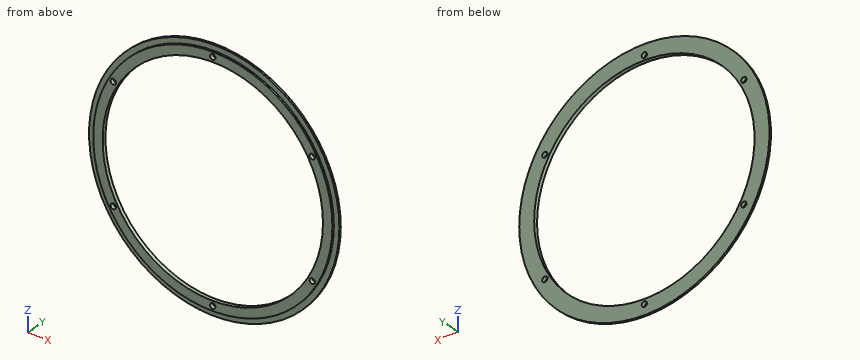
```python
from build123d import *

# Parameters (mm, degrees)
SKETCH1_R           = 160.85
SKETCH1_R_2         = 3.556
SKETCH1_R_3         = 148.15
BOSS_EXTRUDE1_DEPTH = 5.08
SKETCH2_R           = 168.275
SKETCH2_R_2         = 160.85
BOSS_EXTRUDE2_DEPTH = 2.54


with BuildPart() as part:
    # Sketch1 → Boss-Extrude1 (new body)
    with BuildSketch(Plane(origin=(0, 0, 0), x_dir=(1, 0, 0), z_dir=(0, 1, 0))):
        Circle(SKETCH1_R)
        with Locations((0, 154.5)):
            Circle(SKETCH1_R_2, mode=Mode.SUBTRACT)
        with Locations((133.800924885, 77.25)):
            Circle(SKETCH1_R_2, mode=Mode.SUBTRACT)
        with Locations((133.800924885, -77.25)):
            Circle(SKETCH1_R_2, mode=Mode.SUBTRACT)
        with Locations((0, -154.5)):
            Circle(SKETCH1_R_2, mode=Mode.SUBTRACT)
        with Locations((-133.800924885, -77.25)):
            Circle(SKETCH1_R_2, mode=Mode.SUBTRACT)
        with Locations((-133.800924885, 77.25)):
            Circle(SKETCH1_R_2, mode=Mode.SUBTRACT)
        Circle(SKETCH1_R_3, mode=Mode.SUBTRACT)
    extrude(amount=BOSS_EXTRUDE1_DEPTH)

    # Sketch2 → Boss-Extrude2 (add)
    with BuildSketch(Plane(origin=(0, 5.08, 0), x_dir=(1, 0, 0), z_dir=(0, 1, 0))):
        Circle(SKETCH2_R)
        Circle(SKETCH2_R_2, mode=Mode.SUBTRACT)
    extrude(amount=-BOSS_EXTRUDE2_DEPTH)


solid = part.part
```
Can you work these out from the model? Positions are in its coordinate system, mm. Round coordinates to 2 decimals unless told otherwise and drop trailing zeros. Order: outer loops, then holes, each group sorted by start corner. A loop starts at its lowest first (then second) coordinate and runs counter-clockwise, first axis right, second up. Notation, with made-up numbers: (48.5, -31) -> (61.5, -31) arc R29 ccw to (61.5, 0) -> close; hole circle Ø1 at (52, -0.5). An arc over 180 degrees is marked (long way). Return JSON: item names as keys, results as strings. Group by question number.
1. I need wall thicknesses on line 1 (Z direction, x = 0, y = 1.1); line 2 (X direction, y = 1.6, z = -77.25); line 3 (Z direction, x = -134.5, y = 0.75). Which ranges of each line are inside material? Lowest first, please. Write a range as [from, to].
2. If we section it at B-B, the plane y = 3.4: Write out the boundary of the cut face in (x, z) (3 decimals), then the cut area to 3 significant figures.
3. If we section it at C-C, the plane x = -108: Write out the boundary of the cut face in (y, z), then the cut area to 3 significant figures.
4. Will these pins go through, and if not, where does the flat tip stop? pin 1 (2 mm diameter, centred on x = 49, y = 2, fed in from +Z); pin 2 (3 mm diameter, centred on x = 126.5, y = 3.5, fed in from +Z).
5. If we section it at A-A, the plane z = 0: Write out the boundary of the cut face in (x, y) (3 decimals).
Output values:
{
 "1": {"line 1": "[-160.85, -158.06], [-150.94, -148.15], [148.15, 150.94], [158.06, 160.85]", "line 2": "[-141.09, -137.36], [-130.24, -126.42], [126.42, 130.24], [137.36, 141.09]", "line 3": "[-88.22, -80.74], [-73.76, -62.11], [62.11, 73.76], [80.74, 88.22]"},
 "2": {"outline": "circle Ø336.55 at (0, 0); hole circle Ø296.3 at (0, 0); hole circle Ø7.112 at (-133.801, -77.25); hole circle Ø7.112 at (-133.801, 77.25); hole circle Ø7.112 at (0, -154.5); hole circle Ø7.112 at (0, 154.5); hole circle Ø7.112 at (133.801, -77.25); hole circle Ø7.112 at (133.801, 77.25)", "area": "19,800 mm²"},
 "3": {"outline": "(0, -119.2) -> (2.54, -119.2) -> (2.54, -129.04) -> (5.08, -129.04) -> (5.08, -101.41) -> (0, -101.41) -> close; (0, 101.41) -> (5.08, 101.41) -> (5.08, 129.04) -> (2.54, 129.04) -> (2.54, 119.2) -> (0, 119.2) -> close", "area": "231 mm²"},
 "4": {"pin 1": "z = 161.24", "pin 2": "z = 112.66"},
 "5": {"outline": "(-168.275, 2.54) -> (-160.85, 2.54) -> (-160.85, 0) -> (-148.15, 0) -> (-148.15, 5.08) -> (-168.275, 5.08) -> close; (148.15, 0) -> (160.85, 0) -> (160.85, 2.54) -> (168.275, 2.54) -> (168.275, 5.08) -> (148.15, 5.08) -> close"}
}
